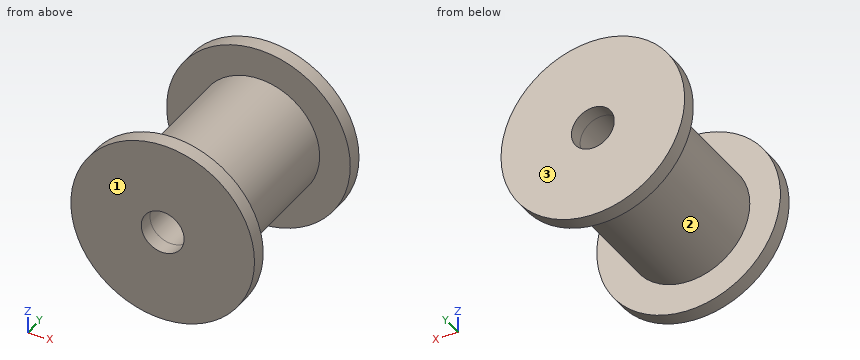
from build123d import *

# Parameters (mm, degrees)
F0_R     = 20
F0_R_2   = 7
F1_DEPTH = 25
F2_R     = 30
F2_R_2   = 7
F3_DEPTH = 5


with BuildPart() as f1:
    # F0 (on Front) → F1 (new body, symmetric)
    with BuildSketch(Plane.XZ):
        Circle(F0_R)
        Circle(F0_R_2, mode=Mode.SUBTRACT)
    extrude(amount=F1_DEPTH, both=True)

    # F2 (on face) → F3 (join)
    with BuildSketch(Plane.XZ.offset(25)):
        Circle(F2_R)
        Circle(F2_R_2, mode=Mode.SUBTRACT)
    extrude(amount=F3_DEPTH)

    # F4: F1 across plane


with BuildPart() as f1_1:
    add(f1.part)
    add(f1.part.mirror(Plane.XZ))


solid = f1_1.part
Part model, mm, in its own coordinate system. Face numbers are marked on the shaded views. Round coordinates to 2 decimals unless told otherwise and drop trailing zeros. Loops run counter-clockwise (first coordinate to the right, second up) from the corner with the lowest first, then second, coordinate; pieces in that order, holes last. Notation, with made-up numbers: (68.25, 70) - (82.25, 70) arc R26 cw to (82.25, 94) - close; hole circle Ø10 at (13, -15.75). An arc over 180 degrees is marked (long way). Answer as a JSON object with one key per item and string values.
Item 1: Band-saw the part on A-A on x = 0. List the corners of the cut face in (y, z), plus the area to 3 significant figures.
Output:
{"outline": "(-30, -30) - (-25, -30) - (-25, -20) - (25, -20) - (25, -30) - (30, -30) - (30, -7) - (-30, -7) - close; (-30, 7) - (30, 7) - (30, 30) - (25, 30) - (25, 20) - (-25, 20) - (-25, 30) - (-30, 30) - close", "area": "1,760 mm2"}
Item 2: Band-saw the part on B-B on z = 0. List the corners of the cut face in (x, y), plus the area to 3 significant figures.
Output:
{"outline": "(-30, -30) - (-7, -30) - (-7, 30) - (-30, 30) - (-30, 25) - (-20, 25) - (-20, -25) - (-30, -25) - close; (7, -30) - (30, -30) - (30, -25) - (20, -25) - (20, 25) - (30, 25) - (30, 30) - (7, 30) - close", "area": "1,760 mm2"}
Item 3: Band-saw the part on C-C on y = -12. List the corners of the cut face in (x, z), plus the area to 3 significant figures.
Output:
{"outline": "circle Ø40 at (0, 0); hole circle Ø14 at (0, 0)", "area": "1,100 mm2"}
Item 4: Pin check, flat tips, straight feed: pin 1 (8 mm diameter, centred on x = -20.5, y = -17, fed in from -Z); pin 2 (4 mm diameter, centred on x = 13.5, y = -18.5, fed in from -Z); pin 3 (1.5 mm diameter, centred on y = 15.5, z = -2, fed in from +X); pin 4 (11 mm diameter, centred on x = 0, z = 0, fed in from +Y). Stop position of each tip, or through.
Output:
{"pin 1": "z = -11.3", "pin 2": "z = -16.36", "pin 3": "x = 19.96", "pin 4": "through"}
Item 5: Band-saw the part on D-D on z = -13. List the corners of the cut face in (x, y), plus the area to 3 significant figures.
Output:
{"outline": "(-27.04, -30) - (27.04, -30) - (27.04, -25) - (15.2, -25) - (15.2, 25) - (27.04, 25) - (27.04, 30) - (-27.04, 30) - (-27.04, 25) - (-15.2, 25) - (-15.2, -25) - (-27.04, -25) - close", "area": "2,060 mm2"}
Item 6: Wall check: L1, parallel to Y at x = 4, z = 26; L2, parallel to Z at x = 0, y = -27; L3, parallel to X at y = 17, z = 0.5. Give the ranges that are in metal, low to high.
Output:
{"L1": "-30 to -25, 25 to 30", "L2": "-30 to -7, 7 to 30", "L3": "-19.99 to -6.98, 6.98 to 19.99"}
Item 7: Pull direction Y, two halves, no side cores. Call the marked faces 1, 2 and 3: pulls with the +Y half, pulls with the -Y half, needs draft (parallel to the pull), parting line crosses it, or undercut.
Output:
{"face 1": "pulls with the -Y half", "face 2": "undercut", "face 3": "pulls with the +Y half"}
